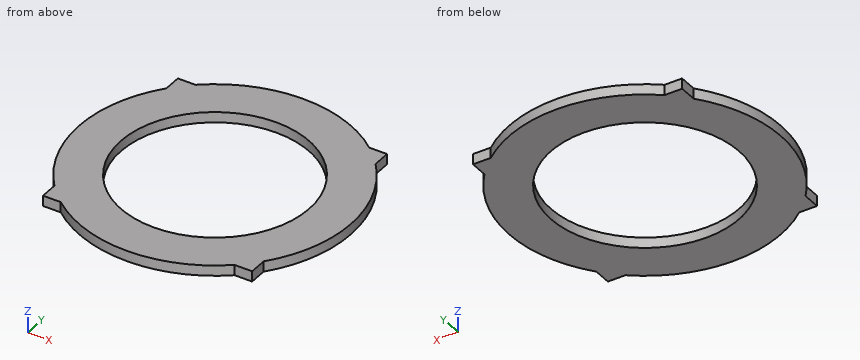
from build123d import *

# Parameters (mm, degrees)
F0_W     = 40
F0_H     = 40
F1_DEPTH = 2
F2_W     = 2
F2_H     = 40
F3_DEPTH = 2
F4_R     = 26
F5_DEPTH = 2
F6_R     = 18
F7_DEPTH = 25


with BuildPart() as f1:
    # F0 (on Top) → F1 (new body)
    with BuildSketch(Plane.XY):
        Rectangle(F0_W, F0_H)
    extrude(amount=F1_DEPTH)

    # F2 (on Top) → F3 (join)
    with BuildSketch(Plane.XY):
        with Locations((-15, 0)):
            Rectangle(F2_W, F2_H)
        with Locations((-11, 0)):
            Rectangle(F2_W, F2_H)
    extrude(amount=F3_DEPTH)

    # F4 (on Top) → F5 (join)
    with BuildSketch(Plane.XY):
        Circle(F4_R)
    extrude(amount=F5_DEPTH)

    # F6 (on face) → F7 (cut)
    with BuildSketch(Plane.XY.offset(2)):
        Circle(F6_R)
    extrude(amount=-F7_DEPTH, mode=Mode.SUBTRACT)


solid = f1.part
Verification items for the finished model (mm, model axes). Coordinates: 2 decimals unless noted, no trailing zeros. Order: outer loops, then holes, each group sorted by start corner. A loop starts at its lowest first (then second) coordinate and runs counter-clockwise, first axis right, second up. Notation, with made-up numbers: M 24.25,83 L 49.25,83 A17 ccw 49.25,110 Z; hole C 3,-11 d1. An arc over 180 degrees is marked long. Write each question's results on one line, items separated by ' | '.
1) Section check C-C on z = 0.3. Record the cut outline in (x, y), plus the area to 3 significant figures.
Solved:
outline: M -20,-20 L -16.61,-20 A26 ccw 16.61,-20 L 20,-20 L 20,-16.61 A26 ccw 20,16.61 L 20,20 L 16.61,20 A26 ccw -16.61,20 L -20,20 L -20,16.61 A26 ccw -20,-16.61 Z; hole C 0,0 d36 | area: 1,130 mm²
2) Gauge pin test, flat ends, axial feed: pin 1 Ø1 at (y, z) = (19, 1) entering from -X; pin 2 Ø1 at (y, z) = (3.5, 1) entering from +X; pin 3 Ø10 at (x, y) = (-8.5, 20) entering from -Z; pin 4 Ø1 at (y, z) = (18.5, 1) entering from +X. Record the tip position at first contact, or that the pin passes through.
Solved:
pin 1: stops at x = -20 | pin 2: stops at x = 25.83 | pin 3: stops at z = 0 | pin 4: stops at x = 20
3) Section check A-A on x = 0. Record the cut outline in (y, z), plus the area to 3 significant figures.
Solved:
outline: M -26,0 L -18,0 L -18,2 L -26,2 Z; M 18,0 L 26,0 L 26,2 L 18,2 Z | area: 32.0 mm²
4) Section check D-D on y = -19. Record the cut outline in (x, z), plus the area to 3 significant figures.
Solved:
outline: M -20,0 L 20,0 L 20,2 L -20,2 Z | area: 80.0 mm²
5) Scan lines: line 1 along Y through (x, z) = (0, 0.6); line 2 along X through (y, z) = (-3, 1.75); line 3 along Y through (x, z) = (-12, 1). Record each from-to range of solid material in increasing order. Write a range as [from, to].
Solved:
line 1: y = [-26, -18], [18, 26] | line 2: x = [-25.83, -17.75], [17.75, 25.83] | line 3: y = [-23.07, -13.42], [13.42, 23.07]
